```python
from build123d import *

# Parameters (mm, degrees)
F0_R     = 101.6
F1_DEPTH = 203.2
F2_T     = -2.54
F4_DEPTH = 127


with BuildPart() as f1:
    # F0 (on Top) → F1 (new body)
    with BuildSketch(Plane.XY):
        Circle(F0_R)
    extrude(amount=F1_DEPTH)

    # F2
    f2_openings = [f1.faces().sort_by_distance(p)[0] for p in [
        (0, 0, 203.2),
    ]]
    offset(amount=F2_T, openings=f2_openings)

    # F3 (on face) → F4 (join)
    with BuildSketch(Plane(origin=(0, 0, 0), x_dir=(1, 0, 0), z_dir=(0, 0, -1))):
        with BuildLine():
            ThreePointArc((-49.356736, 88.805814), (-48.279072, 89.39626), (-47.194345, 89.973629))
            Line((-47.194345, 89.973629), (-49.356736, 89.973629))
            Line((-49.356736, 89.973629), (-49.356736, 88.805814))
        make_face()
        with BuildLine():
            Line((19.613178, 21.691842), (19.613178, 89.973629))
            Line((19.613178, 89.973629), (-47.194345, 89.973629))
            ThreePointArc((-47.194345, 89.973629), (-48.279072, 89.39626), (-49.356736, 88.805814))
            Line((-49.356736, 88.805814), (-49.356736, 21.691842))
            Line((-49.356736, 21.691842), (19.613178, 21.691842))
        make_face()
    extrude(amount=F4_DEPTH)


solid = f1.part
```
Geometry: final body of the model. Coordinates: model frame, mm. A direction names the side the tool comes from. Coordinates: 2 decimals unless noted, no trailing zeros. Order: outer loops, then holes, each group sorted by start corner. A loop starts at its lowest first (then second) coordinate and runs counter-clockwise, first axis right, second up.
Item 1: Section query C-C (z = 145.5). Output: boundary loops of the cut face in (x, y), then the cut area to 3 significant figures.
Answer:
outline: circle Ø203.2 at (0, 0); hole circle Ø198.12 at (0, 0)
area: 1,600 mm2
Item 2: Draft query along Y for faces 4 (the face through (-1, 1, 2.54)), 5 (the face through (-14, -89.974, -63)), 6 (the face through (19.613, -55, -63)), 7 (the face through (-15, -21.692, -63)). Return one class per face: released by +Y, released by -Y, zero draft, split by the parting line, or undercut.
Answer:
face 4: undercut
face 5: released by -Y
face 6: zero draft
face 7: released by +Y
Item 3: Section query D-D (z = -103). Output: boundary loops of the cut face in (x, y).
Answer:
outline: (-49.36, -89.97) - (19.61, -89.97) - (19.61, -21.69) - (-49.36, -21.69) - close
Item 4: Contact query for flat-ended pins moving along their axis: P1, Ø12, axis at x = 56, y = 38, coming from the -Z side; P2, Ø5, axis at y = -31.5, z = 4, coming from the +X side; P3, Ø5, axis at x = 48.5, z = 110.5, coming from the +Y side. Output: stop coordinate, or through.
Answer:
P1: stops at z = 0
P2: stops at x = 97.37
P3: stops at y = 90.59
Item 5: Material intervals for line 1 along Y through (x, z) = (0, 121); line 2 along Z through (x, y) = (-7.5, 86), sorted ascending.
Answer:
line 1: y = -101.6 to -99.06, 99.06 to 101.6
line 2: z = 0 to 2.54
Item 6: Section query A-A (x = 0). Output: boundary loops of the cut face in (y, z).
Answer:
outline: (-101.6, 0) - (-89.97, 0) - (-89.97, -127) - (-21.69, -127) - (-21.69, 0) - (101.6, 0) - (101.6, 203.2) - (99.06, 203.2) - (99.06, 2.54) - (-99.06, 2.54) - (-99.06, 203.2) - (-101.6, 203.2) - close
Item 7: Access query for faces 1 (the face through (-15, -56, -127)), 2 (the face through (-12.896, 98.217, 101.465)), 3 (the face through (-49.357, -56, -63)). Directions: +Z, -Z, +X, -X, +Y, -Y. A direction counts if a zero-diameter tool reaches every point of the face in a straight line with its end or side. Return the directions, or none.
Answer:
face 1: -Z, +X, -X, +Y, -Y
face 2: +Z
face 3: -Z, -X, +Y, -Y
Item 8: Section query B-B (y = 0). Output: boundary loops of the cut face in (x, z), then the cut area to 3 significant figures.
Answer:
outline: (-101.6, 0) - (101.6, 0) - (101.6, 203.2) - (99.06, 203.2) - (99.06, 2.54) - (-99.06, 2.54) - (-99.06, 203.2) - (-101.6, 203.2) - close
area: 1,540 mm2
